```python
from build123d import *

# Parameters (mm, degrees)
F1_DEPTH    = 920
F2_T1_DEPTH = 47.7168298797
F4_DEPTH    = 25
F5_T1_DEPTH = 47.7168298797
F7_DEPTH    = 25


# Not quite as in the source:
# - a fillet or chamfer that OpenCascade refuses, or shapes differently, is made with other operations: its cross-section is extruded or revolved along the edge and cut away or added


with BuildPart() as f1:
    # F0 (on Front) → F1 (new body)
    with BuildSketch(Plane.XZ):
        Polygon((0, 3), (0, 0), (25, 0), (25, 25), (22, 25), (22, 3), align=None)
    extrude(amount=F1_DEPTH)

    # F2: chamfer of 5 on 1 edges, made by hand

    # F2_s2 → F2_t1 (cut)
    with BuildSketch(Plane.XY.offset(-9.8584149398)):
        Polygon((22, -5), (27, 0), (22, 0), align=None)
    extrude(amount=F2_T1_DEPTH, mode=Mode.SUBTRACT)

    # F3 (on face) → F4 (cut)
    with BuildSketch(Plane.XY.offset(3)):
        Polygon((0, -27), (22, -5), (22, 0), (0, 0), align=None)
    extrude(amount=-F4_DEPTH, mode=Mode.SUBTRACT)

    # F5: chamfer of 5 on 1 edges, made by hand

    # F5_s2 → F5_t1 (cut)
    with BuildSketch(Plane.XY.offset(-9.8584149398)):
        Polygon((22, -915), (27, -920), (22, -920), align=None)
    extrude(amount=F5_T1_DEPTH, mode=Mode.SUBTRACT)

    # F6 (on face) → F7 (cut)
    with BuildSketch(Plane.XY.offset(3)):
        Polygon((22, -920), (22, -915), (0, -893), (0, -920), align=None)
    extrude(amount=-F7_DEPTH, mode=Mode.SUBTRACT)


solid = f1.part
```
Design review of the part built by this model. Coordinates are the model's own, in mm. A direction names the side the tool comes from. Coordinates: 2 decimals unless noted, no trailing zeros. Order: outer loops, then holes, each group sorted by start corner. A loop starts at its lowest first (then second) coordinate and runs counter-clockwise, first axis right, second up. Notation, with made-up numbers: (88.25, 20) - (125.25, 20) arc R29 ccw to (125.25, 54) - close; hole circle Ø7 at (21, 1.5). An arc over 180 degrees is marked (long way). Answer in a Markdown table with one row per item.
(1) Consider section C-C on y = -855.5. State the section outline as (x, z) points, plus the area to 3 significant figures.
Checked values:
| item | result |
|---|---|
| outline | (0, 0) - (25, 0) - (25, 25) - (22, 25) - (22, 3) - (0, 3) - close |
| area | 141 mm^2 |
(2) Consider section A-A on x = 4.25. State the section outline as (y, z) points, plus the area to 3 significant figures.
Checked values:
| item | result |
|---|---|
| outline | (-897.25, 0) - (-22.75, 0) - (-22.75, 3) - (-897.25, 3) - close |
| area | 2,620 mm^2 |
(3) Clearance check with a flat-ended pin moving along its axis: pin 1 (5 mm diameter, centred on y = -205.5, z = 15, fed in from -X). State where the tip first meets the part, or that it passes through.
Checked values:
| item | result |
|---|---|
| pin 1 | x = 22 |
(4) For faces 1 (the flat face through (22, -454, 14)), 2 (the flat face through (25, -454, 12)), list the 3-axis set-ups (+Z, -Z, +X, -X, +Y, -Y) from which the entire face can be reached by the end or side of a thin tool; tool diameter is ignored.
Checked values:
| item | result |
|---|---|
| face 1 | +Z, -X, +Y, -Y |
| face 2 | +Z, -Z, +X, +Y, -Y |
(5) Wall thickness on line 1 along Z through (x, y) = (19, -127); line 2 along X through (y, z) = (-116, 22.5); line 3 along Y through (x, z) = (24, 8): over which ranges is each line inside the solid? List them lowest first. Write a range as from..to.
Checked values:
| item | result |
|---|---|
| line 1 | 0..3 |
| line 2 | 22..25 |
| line 3 | -917..-3 |
(6) Consider section B-B on z = 13.75. State the section outline as (x, y) points.
Checked values:
| item | result |
|---|---|
| outline | (22, -915) - (25, -918) - (25, -2) - (22, -5) - close |
